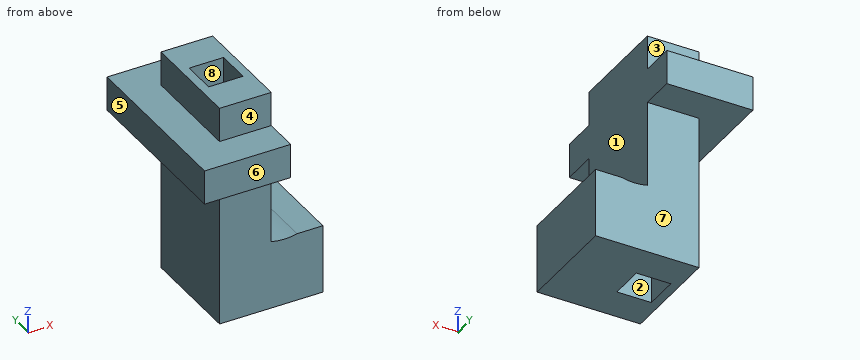
```python
from build123d import *

# Parameters (mm, degrees)
F0_W      = 38.1
F0_H      = 76.2
F1_DEPTH  = 177.8
F2_W      = 76.2
F2_H      = 25.4
F3_DEPTH  = 25.4
F5_DEPTH  = 25.4
F7_DEPTH  = 25.4
F9_W      = 38.1
F9_H      = 76.2
F10_DEPTH = 25.4
F11_W     = 25.4
F11_H     = 25.4
F12_DEPTH = 228.6
F13_W     = 76.2
F13_H     = 50.8
F14_DEPTH = 38.1
F16_DEPTH = 228.6
F17_W     = 38.1
F17_H     = 76.2
F17_W_2   = 25.4
F17_H_2   = 25.4
F18_DEPTH = 38.1


with BuildPart() as f1:
    # F0 (on Top) → F1 (new body)
    with BuildSketch(Plane.XY):
        Rectangle(F0_W, F0_H)
    extrude(amount=F1_DEPTH)

    # F2 (on face) → F3 (join)
    with BuildSketch(Plane(origin=(-19.05, 0, 0), x_dir=(0, -1, 0), z_dir=(-1, 0, 0))):
        with Locations((0, 127)):
            Rectangle(F2_W, F2_H)
    extrude(amount=F3_DEPTH)

    # F4 (on face) → F5 (join)
    with BuildSketch(Plane.XZ.offset(38.1)):
        Polygon((-44.45, 139.7), (-44.45, 114.3), (-19.05, 114.3), (19.05, 114.3), (19.05, 139.7), (-19.05, 139.7), align=None)
    extrude(amount=F5_DEPTH)

    # F6 (on face) → F7 (join)
    with BuildSketch(Plane(origin=(0, 38.1, 0), x_dir=(-1, 0, 0), z_dir=(0, 1, 0))):
        Polygon((44.45, 114.3), (44.45, 139.7), (19.05, 139.7), (-19.05, 139.7), (-19.05, 114.3), (19.05, 114.3), align=None)
    extrude(amount=F7_DEPTH)

    # F9 (on face) → F10 (join)
    with BuildSketch(Plane.XY.offset(177.8)):
        Rectangle(F9_W, F9_H)
    extrude(amount=F10_DEPTH)

    # F11 (on face) → F12 (cut)
    with BuildSketch(Plane.XY.offset(203.2)):
        Rectangle(F11_W, F11_H)
    extrude(amount=-F12_DEPTH, mode=Mode.SUBTRACT)

    # F13 (on face) → F14 (join)
    with BuildSketch(Plane.YZ.offset(19.05)):
        with Locations((0, 25.4)):
            Rectangle(F13_W, F13_H)
    extrude(amount=F14_DEPTH)

    # F15 (on face) → F16 (cut)
    with BuildSketch(Plane.XZ.offset(38.1)):
        with BuildLine():
            Line((38.1, 50.8), (19.05, 50.8))
            ThreePointArc((19.05, 50.8), (28.575, 49.5901663726), (38.1, 50.8))
        make_face()
    extrude(amount=-F16_DEPTH, mode=Mode.SUBTRACT)

    # F17 (on face) → F18 (cut)
    with BuildSketch(Plane.XY.offset(203.2)):
        Rectangle(F17_W, F17_H)
        Rectangle(F17_W_2, F17_H_2, mode=Mode.SUBTRACT)
    extrude(amount=-F18_DEPTH, mode=Mode.SUBTRACT)


solid = f1.part
```
Model file for the job. Use its own axes, mm. Face numbers are marked on the shaded views. A direction names the side the tool comes from. Coordinates: 2 decimals unless noted, no trailing zeros. Loops run counter-clockwise (first coordinate to the right, second up) from the corner with the lowest first, then second, coordinate; pieces in that order, holes last. Notation, with made-up numbers: (58, -6.75) -> (69, -6.75) arc R10 ccw to (69, 1.25) -> close; hole circle Ø8 at (-18.75, 85). An arc over 180 degrees is marked (long way). Answer as a JSON object with one key per item and string values.
Q1. Probe probe 1 along Y at (x, z) = (-7, 116.5); probe 2 along X at (y, z) = (-9, 125); probe 3 along X at (y, z) = (-0.5, 97.5). List the from-to ranges inside material, lowest first.
Report:
{"probe 1": "y = -63.5 to -12.7, 12.7 to 63.5", "probe 2": "x = -44.45 to -12.7, 12.7 to 19.05", "probe 3": "x = -19.05 to -12.7, 12.7 to 19.05"}
Q2. Cut at B-B (y = 1). List the corners of the cut face in (x, z) (3 decimals), and give its area (3 significant figures).
Report:
{"outline": "(-44.45, 114.3) -> (-19.05, 114.3) -> (-19.05, 0) -> (-12.7, 0) -> (-12.7, 165.1) -> (-19.05, 165.1) -> (-19.05, 139.7) -> (-44.45, 139.7) -> close; (12.7, 0) -> (57.15, 0) -> (57.15, 50.8) -> (38.1, 50.8) arc R38.1 cw to (19.05, 50.8) -> (19.05, 165.1) -> (12.7, 165.1) -> close", "area": "4,660 mm2"}
Q3. Cut at A-A (z = 36). List the corners of the cut face in (x, y), and give its area (3 significant figures).
Report:
{"outline": "(-19.05, -38.1) -> (57.15, -38.1) -> (57.15, 38.1) -> (-19.05, 38.1) -> close; hole (-12.7, -12.7) -> (12.7, -12.7) -> (12.7, 12.7) -> (-12.7, 12.7) -> close", "area": "5,160 mm2"}
Q4. Cut at C-C (x = 16). List the corners of the cut face in (y, z), and give its area (3 significant figures).
Report:
{"outline": "(-63.5, 114.3) -> (-38.1, 114.3) -> (-38.1, 0) -> (38.1, 0) -> (38.1, 114.3) -> (63.5, 114.3) -> (63.5, 139.7) -> (38.1, 139.7) -> (38.1, 165.1) -> (-38.1, 165.1) -> (-38.1, 139.7) -> (-63.5, 139.7) -> close", "area": "13,900 mm2"}
Q5. Pull direction Y, two halves, no side cores. Call the marked faces 5, 6, 7 and 8: released by +Y, released by -Y, zero draft, split by the parting line, or undercut.
Report:
{"face 5": "zero draft", "face 6": "released by -Y", "face 7": "released by +Y", "face 8": "undercut"}
Q6. Flat gauge pins, fed straight in: P1, Ø12.5, axis at x = -0.5, z = 88.5, coming from the -Y side; P2, Ø12.5, axis at y = 17.5, z = 148, coming from the -X side; P3, Ø6, axis at x = -31.5, y = 27, coming from the +Z side. Where does each tip first touch, or does it go through?
Report:
{"P1": "stops at y = -38.1", "P2": "stops at x = -19.05", "P3": "stops at z = 139.7"}
Q7. 3-axis set-ups, long thin cutter, end or side, ignore diameter. For the marked faces 1, 2, 3 and 4: which of +Z, -Z, +X, -X, +Y, -Y reach the whole face in a straight line?
Report:
{"face 1": "+Z, +X, +Y, -Y", "face 2": "+Z, -Z", "face 3": "+Z, +X, -X, +Y", "face 4": "+Z, +X, -X, -Y"}
Q8. Cut at D-D (z = 127). List the corners of the cut face in (x, y).
Report:
{"outline": "(-44.45, -63.5) -> (19.05, -63.5) -> (19.05, 63.5) -> (-44.45, 63.5) -> close; hole (-12.7, -12.7) -> (12.7, -12.7) -> (12.7, 12.7) -> (-12.7, 12.7) -> close"}
